```python
from build123d import *

# Parameters (mm, degrees)
EXTRUDE_1_DEPTH     = 100
CUT_EXTRUDE_1_DEPTH = 100
SKETCH_5_W          = 43.975139672
SKETCH_5_H          = 100.104675822
CUT_EXTRUDE_3_DEPTH = 8


with BuildPart() as part:
    # 草图2 → 凸台-拉伸1 (new body)
    with BuildSketch(Plane.XY):
        with BuildLine():
            Line((0, 20), (80, 20))
            Line((80, 20), (80, -20))
            Line((80, -20), (0, -20))
            ThreePointArc((0, -20), (-20, 0), (0, 20))
        make_face()
    extrude(amount=EXTRUDE_1_DEPTH)

    # 草图3 → 切除-拉伸1 (cut)
    with BuildSketch(Plane(origin=(0, 20, 0), x_dir=(1, 0, 0), z_dir=(0, 1, 0))):
        with BuildLine():
            Line((40, 0), (74.482758502, -36.206896811))
            ThreePointArc((74.482758502, -36.206896811), (79.999999735, -50), (74.482758502, -63.793103189))
            Line((74.482758502, -63.793103189), (40, -100))
            Line((40, -100), (91.714369415, -100))
            Line((91.714369415, -100), (91.714369415, 0))
            Line((91.714369415, 0), (40, 0))
        make_face()
    extrude(amount=-CUT_EXTRUDE_1_DEPTH, mode=Mode.SUBTRACT)

    # 草图5 → 切除-拉伸3 (cut, symmetric)
    with BuildSketch(Plane(origin=(0, 0, 0), x_dir=(1, 0, 0), z_dir=(0, 1, 0))):
        with Locations((61.987569836, -50.052337911)):
            Rectangle(SKETCH_5_W, SKETCH_5_H)
    extrude(amount=CUT_EXTRUDE_3_DEPTH, both=True, mode=Mode.SUBTRACT)


solid = part.part
```
The model under review builds one solid part; all positions refer to its coordinate system, in mm. A direction names the side the tool comes from. Coordinates: 2 decimals unless noted, no trailing zeros. Write each loop counter-clockwise with the first axis right and the second up, starting at its lowest first coordinate (ties: lowest second). Pieces come first, ordered by that corner, then holes. Notation, with made-up numbers: (-37, 52.25) - (8, 52.25) arc R21 cw to (8, 66.25) - close; hole circle Ø6 at (66.25, 78.5). An arc over 180 degrees is marked (long way). Write item = value, one per line.
(1) Consider section C-C, the plane y = 16. Give the boundary of the cut face in (x, z), then the cut area to 3 significant figures.
Result sheet:
outline = (-12, 0) - (40, 0) - (74.48, 36.21) arc R20 ccw to (74.48, 63.79) - (40, 100) - (-12, 100) - close
area = 7,500 mm^2
(2) For P1, Ø3, axis at x = 51.5, y = 11, coming from the -Z side; P2, Ø8, axis at y = 0, z = 70.5, coming from the +X side; P3, Ø1, axis at y = -13.5, z = 86.5, coming from the -X side, all flat-tipped, find the tip position at first contact; note any pin that passes through.
Result sheet:
P1 = 10.5
P2 = 40
P3 = -15.2
(3) Consider section A-A, the plane x = 46. Give the boundary of the cut face in (y, z).
Result sheet:
outline = (-20, 6.3) - (-8, 6.3) - (-8, 93.7) - (-20, 93.7) - close; (8, 6.3) - (20, 6.3) - (20, 93.7) - (8, 93.7) - close
(4) Consider section B-B, the plane z = 59.5. Give the boundary of the cut face in (x, y), then the cut area to 3 significant figures.
Result sheet:
outline = (0, -20) - (77.6, -20) - (77.6, -8) - (40, -8) - (40, 8) - (77.6, 8) - (77.6, 20) - (0, 20) arc R20 ccw to start
area = 3,130 mm^2
(5) For line 1 (Y direction, x = 44, z = 49.5); line 2 (X direction, y = 1, z = 17.5); line 3 (X direction, y = -3.5, z = 42), list the stretches that pass through material, from the lowest coordinate up. Write a range as [from, to].
Result sheet:
line_1 = [-20, -8], [8, 20]
line_2 = [-19.97, 40]
line_3 = [-19.69, 40]
(6) Consider section D-D, the plane x = 67.5. Give the boundary of the cut face in (y, z) (3 decimals), then the cut area to 3 significant figures.
Result sheet:
outline = (-20, 28.875) - (-8, 28.875) - (-8, 71.125) - (-20, 71.125) - close; (8, 28.875) - (20, 28.875) - (20, 71.125) - (8, 71.125) - close
area = 1,010 mm^2
(7) Machinability: for faces 1 (the face through (55, -8, 49)), 2 (the face through (57, 14.08, 17.85)), which of the approach directions +Z, -Z, +X, -X, +Y, -Y give a long, thin tool a straight path to every point of the face, cutting with its end or side? Answer none if there is none.
Result sheet:
face_1 = +Z, -Z, +X
face_2 = -Z, +X, +Y, -Y
